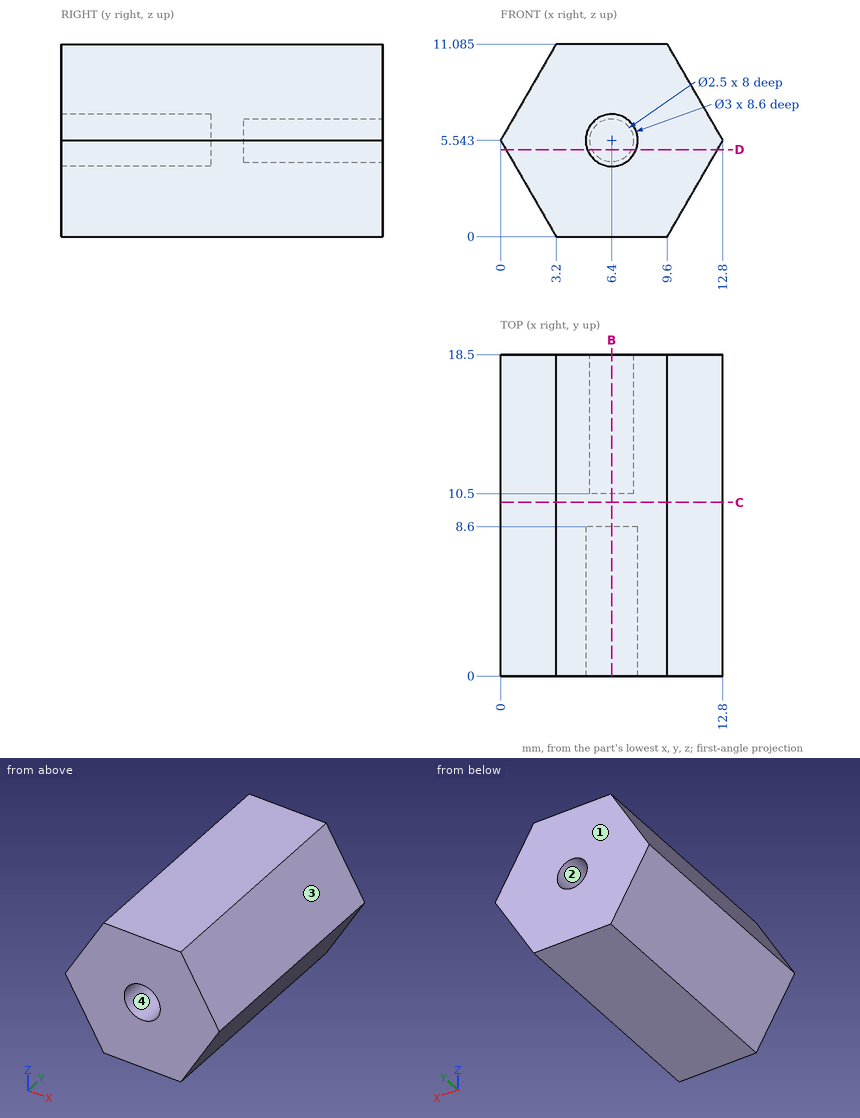
The figure shows three views and two pictorial views of one solid part (mm, origin at its lowest corner). Answer the questions. Round coordinates to 2 decimals unless told otherwise and drop trailing zeros. Write each loop counter-clockwise with the first axis right and the second up, starting at its lowest first coordinate (ties: lowest second). Pieces come first, ordered by that corner, then holes. Notation, with made-up numbers: M 72.25,52.5 L 111.25,52.5 A18 cw 111.25,60.5 Z; hole C -20.5,-18.75 d4. An arc over 180 degrees is marked long. Use a Markdown table: item, result.
1) For a pull along X with two mould halves and no side action, classify the marked faces 1, 2, 3 and 4 as pulls with the +X half, pulls with the -X half, needs draft (parallel to the pull), parting line crosses it, or undercut.
Answers follow:
| item | result |
|---|---|
| face 1 | needs draft |
| face 2 | undercut |
| face 3 | pulls with the +X half |
| face 4 | undercut |
2) The part is cut by section C-C (y = 10). Write down the section's boundary in (x, z) (1 decimal).
Answers follow:
| item | result |
|---|---|
| outline | M 0,5.5 L 3.2,0 L 9.6,0 L 12.8,5.5 L 9.6,11.1 L 3.2,11.1 Z |
3) Flat-ended cylindrical pins translate along their axes: pin 1 (2 mm diameter, centred on x = 6.4, z = 5.54, fed in from -Y); pin 2 (1 mm diameter, centred on y = 8.5, z = 4, fed in from -X); pin 3 (3 mm diameter, centred on y = 4.5, z = 8.5, fed in from -X). Find the tip coordinate at first contact, or state that the pin passes through.
Answers follow:
| item | result |
|---|---|
| pin 1 | stops at y = 8.6 |
| pin 2 | stops at x = 0.6 |
| pin 3 | stops at x = 0.84 |
4) The part is cut by section D-D (z = 5). Write down the section's boundary in (x, y).
Answers follow:
| item | result |
|---|---|
| outline | M 0.31,0 L 5,0 L 5,8.6 L 7.8,8.6 L 7.8,0 L 12.49,0 L 12.49,18.5 L 7.53,18.5 L 7.53,10.5 L 5.27,10.5 L 5.27,18.5 L 0.31,18.5 Z |
5) Straight lines are drawn through the part: line 1 along Z through (x, y) = (6.4, 12.25) (1 decimal); line 2 along Z through (x, y) = (6.4, 6.25) (1 decimal); line 3 along X through (y, z) = (16.25, 6) (1 decimal). For each, find the intervals that lie inside material, in ascending order. Write a range as [from, to].
Answers follow:
| item | result |
|---|---|
| line 1 | z = [0, 4.3], [6.8, 11.1] |
| line 2 | z = [0, 4], [7, 11.1] |
| line 3 | x = [0.3, 5.2], [7.6, 12.5] |
6) The part is cut by section B-B (x = 6.4). Write down the section's boundary in (y, z) (1 decimal), plus the area to 3 significant figures.
Answers follow:
| item | result |
|---|---|
| outline | M 0,0 L 18.5,0 L 18.5,4.3 L 10.5,4.3 L 10.5,6.8 L 18.5,6.8 L 18.5,11.1 L 0,11.1 L 0,7 L 8.6,7 L 8.6,4 L 0,4 Z |
| area | 159 mm2 |
